Read the model definition and answer for the solid it produces. Units are mm, in the model's axes. A direction names the side the tool comes from. Give positions to 0.01 mm unless a question says otherwise; leave off trailing zeros. Order: outer loops, then holes, each group sorted by start corner. A loop starts at its lowest first (then second) coordinate and runs counter-clockwise, first axis right, second up.
```python
from build123d import *

# Parameters (mm, degrees)
SKETCH_1_R        = 13.4
SKETCH_1_R_2      = 4.5
D26P8H18P5_DEPTH  = 16.5
EXTRUDE_START     = 15
SKETCH_2_R        = 13.4
EXTRUDE_292_DEPTH = 1.5
EXTRUDE_START_2   = -2
SKETCH_3_R        = 11
EXTRUDE_347_DEPTH = 2
EXTRUDE_START_3   = 16.5
SKETCH_4_R        = 2.5
EXTRUDE_M5_DEPTH  = 12.3
D16_M3_START      = -2
SKETCH_5_R        = 1.6
D16_M3_DEPTH      = 5


with BuildPart() as part:
    # 草图1 → 钟罩及定子总包络_D26p8H18p5 (new body)
    with BuildSketch(Plane.XY):
        Circle(SKETCH_1_R)
        Circle(SKETCH_1_R_2, mode=Mode.SUBTRACT)
    extrude(amount=D26P8H18P5_DEPTH)

    # 草图2 → Extrude 292 (add)
    with BuildSketch(Plane.XY.offset(EXTRUDE_START)):
        Circle(SKETCH_2_R)
    extrude(amount=EXTRUDE_292_DEPTH)

    # 草图3 → Extrude 347 (add)
    with BuildSketch(Plane.XY.offset(EXTRUDE_START_2)):
        Circle(SKETCH_3_R)
    extrude(amount=EXTRUDE_347_DEPTH)

    # 草图4 → M5桨轴包络 (add)
    with BuildSketch(Plane.XY.offset(EXTRUDE_START_3)):
        Circle(SKETCH_4_R)
    extrude(amount=EXTRUDE_M5_DEPTH)

    # 草图5 → D16分度圆四M3简化安装孔 (cut)
    with BuildSketch(Plane.XY.offset(D16_M3_START)):
        with Locations((-8, 0)):
            Circle(SKETCH_5_R)
        with Locations((0, -8)):
            Circle(SKETCH_5_R)
        with Locations((8, 0)):
            Circle(SKETCH_5_R)
        with Locations((0, 8)):
            Circle(SKETCH_5_R)
    extrude(amount=D16_M3_DEPTH, mode=Mode.SUBTRACT)


solid = part.part
```
1) Given pin 1 (2.5 mm diameter, centred on x = 0, y = -8, fed in from -Z); pin 2 (3 mm diameter, centred on x = 8, y = 0, fed in from +Z); pin 3 (12 mm diameter, centred on y = 8, z = 20.5, fed in from +X), each flat-ended and moving along its own axis, determine where each tip first touches the part or whether it passes through.
Final values:
pin 1: stops at z = 3
pin 2: stops at z = 16.5
pin 3: stops at x = 12.93
2) The part is cut by section D-D on x = -8. Determine the outline of the cut face in (y, z).
Final values:
outline: (-10.75, 0) - (-7.55, 0) - (-7.55, -2) - (-1.6, -2) - (-1.6, 3) - (1.6, 3) - (1.6, -2) - (7.55, -2) - (7.55, 0) - (10.75, 0) - (10.75, 16.5) - (-10.75, 16.5) - close
3) The part is cut by section A-A on x = 0. Determine the outline of the cut face in (y, z).
Final values:
outline: (-13.4, 0) - (-11, 0) - (-11, -2) - (-9.6, -2) - (-9.6, 3) - (-6.4, 3) - (-6.4, -2) - (6.4, -2) - (6.4, 3) - (9.6, 3) - (9.6, -2) - (11, -2) - (11, 0) - (13.4, 0) - (13.4, 16.5) - (2.5, 16.5) - (2.5, 28.8) - (-2.5, 28.8) - (-2.5, 16.5) - (-13.4, 16.5) - close; hole (-4.5, 0) - (4.5, 0) - (4.5, 15) - (-4.5, 15) - close
4) For a pull along Z with two mould halves and no side action, classify faces 6 (the face through (-9.6, 0.07, 0.46)), 7 (the face through (0, 0, 0)), 8 (the face through (8, 0, 3)) as released by +Z, released by -Z, zero draft, split by the parting line, or undercut.
Final values:
face 6: zero draft
face 7: undercut
face 8: released by -Z
5) The part is cut by section C-C on z = 12. Determine the outline of the cut face in (x, y).
Final values:
outline: circle Ø26.8 at (0, 0); hole circle Ø9 at (0, 0)
6) A tool of negligible diameter and unlimited length cuts with its end or side. For faces 1 (the face through (0, 0, 28.8)), 2 (the face through (-13.387, 0.589, 8.134)), 3 (the face through (-0.59, 4.46, 7.4)), 4 (the face through (0, 8, 3)), 5 (the face through (-0.54, -2.44, 22.56)), from which of +Z, -Z, +X, -X, +Y, -Y can it reach the whole face along a straight path? Write none if from no direction.
Final values:
face 1: +Z, +X, -X, +Y, -Y
face 2: +Z, -Z
face 3: none
face 4: -Z
face 5: +Z
7) Consider L1, parallel to Y at x = 0, z = 0.2; L2, parallel to Z at x = 5, y = -2; L3, parallel to Z at x = 2.75, y = -12. Determine where each line is inside the solid, lowest interval first.
Final values:
L1: y = -13.4 to -9.6, -6.4 to -4.5, 4.5 to 6.4, 9.6 to 13.4
L2: z = -2 to 16.5
L3: z = 0 to 16.5
